```python
from build123d import *

# Parameters (mm, degrees)
BOSS_EXTRU_1_DEPTH      = 120
ENL_V_MAT_EXTRU_1_DEPTH = 188.009777727
ENL_V_MAT_EXTRU_2_DEPTH = 180.784310366
ESQUISSE6_R             = 2
ENL_V_MAT_EXTRU_3_DEPTH = 188.009777727
ESQUISSE7_R             = 2
ENL_V_MAT_EXTRU_4_DEPTH = 180.784310366
ESQUISSE10_R            = 1.364499713
ENL_V_MAT_EXTRU_5_DEPTH = 180.784310366
ENL_V_MAT_EXTRU_6_DEPTH = 188.009777727
ESQUISSE11_R            = 2
ENL_V_MAT_EXTRU_7_DEPTH = 188.009777727
ESQUISSE12_R            = 2
ENL_V_MAT_EXTRU_8_DEPTH = 180.784310366


with BuildPart() as part:
    # Esquisse3 → Boss.-Extru.1 (new body)
    with BuildSketch(Plane(origin=(0, 0, 0), x_dir=(1, 0, 0), z_dir=(0, 1, 0))):
        with BuildLine():
            ThreePointArc((-25, -28.618176043), (-27.104360033, -26.633694209), (-29.051678093, -24.494897428))
            Line((-29.051678093, -24.494897428), (-115, -24.494897428))
            Line((-115, -24.494897428), (-115, -28.618176043))
            Line((-115, -28.618176043), (-25, -28.618176043))
        make_face()
        with BuildLine():
            ThreePointArc((-10.103808925, -33.509894736), (-18.121448463, -29.943498553), (-25, -24.494897428))
            Line((-25, -24.494897428), (-29.051678093, -24.494897428))
            ThreePointArc((-29.051678093, -24.494897428), (-27.104360033, -26.633694209), (-25, -28.618176043))
            ThreePointArc((-25, -28.618176043), (-19.581111, -32.566548666), (-13.552631037, -35.50107311))
            ThreePointArc((-13.552631037, -35.50107311), (-10.809506446, -36.430132725), (-8.003591765, -37.147577564))
            Line((-8.003591765, -37.147577564), (-10.103808925, -33.509894736))
        make_face()
        with BuildLine():
            Line((35.411933246, -112.345472721), (-8.003591765, -37.147577564))
            ThreePointArc((-8.003591765, -37.147577564), (-10.809506446, -36.430132725), (-13.552631037, -35.50107311))
            Line((-13.552631037, -35.50107311), (31.963111135, -114.336651096))
            Line((31.963111135, -114.336651096), (35.411933246, -112.345472721))
        make_face()
    extrude(amount=BOSS_EXTRU_1_DEPTH)

    # Esquisse4 → Enlèv. mat.-Extru.1 (cut, through all)
    with BuildSketch(Plane.XY.offset(28.618176043)):
        with BuildLine():
            Line((-48, 105), (-48, 15))
            ThreePointArc((-48, 15), (-40, 7), (-32, 15))
            Line((-32, 15), (-32, 105))
            ThreePointArc((-32, 105), (-40, 113), (-48, 105))
        make_face()
    extrude(amount=-ENL_V_MAT_EXTRU_1_DEPTH, mode=Mode.SUBTRACT)

    # Esquisse5 → Enlèv. mat.-Extru.2 (cut, through all)
    with BuildSketch(Plane(origin=(-25.536888865, 0, 14.743729661), x_dir=(0.4999999999999999, 0, 0.8660254037844386), z_dir=(-0.8660254037844387, 0, 0.49999999999999994))):
        with BuildLine():
            Line((46.968515657, 105), (46.968515657, 15))
            ThreePointArc((46.968515657, 15), (38.968515657, 7), (30.968515657, 15))
            Line((30.968515657, 15), (30.968515657, 105))
            ThreePointArc((30.968515657, 105), (38.968515657, 113), (46.968515657, 105))
        make_face()
    extrude(amount=-ENL_V_MAT_EXTRU_2_DEPTH, mode=Mode.SUBTRACT)

    # Esquisse6 → Enlèv. mat.-Extru.3 (cut, through all)
    with BuildSketch(Plane.XY.offset(28.618176043)):
        with Locations((-110, 106.75)):
            Circle(ESQUISSE6_R)
    extrude(amount=-ENL_V_MAT_EXTRU_3_DEPTH, mode=Mode.SUBTRACT)

    # Esquisse7 → Enlèv. mat.-Extru.4 (cut, through all)
    with BuildSketch(Plane(origin=(-25.536888865, 0, 14.743729661), x_dir=(0.4999999999999999, 0, 0.8660254037844386), z_dir=(-0.8660254037844387, 0, 0.49999999999999994))):
        with Locations((110, 106.75)):
            Circle(ESQUISSE7_R)
    extrude(amount=-ENL_V_MAT_EXTRU_4_DEPTH, mode=Mode.SUBTRACT)

    # Esquisse10 → Enlèv. mat.-Extru.5 (cut, through all)
    with BuildSketch(Plane(origin=(-25.536888865, 0, 14.743729661), x_dir=(0.4999999999999999, 0, 0.8660254037844386), z_dir=(-0.8660254037844387, 0, 0.49999999999999994))):
        with Locations((101.5, 23.5)):
            Circle(ESQUISSE10_R)
        with Locations((52.5, 23.5)):
            Circle(ESQUISSE10_R)
        with Locations((52.5, 81.585512482)):
            Circle(ESQUISSE10_R)
        with Locations((101.5, 81.585512482)):
            Circle(ESQUISSE10_R)
    extrude(amount=-ENL_V_MAT_EXTRU_5_DEPTH, mode=Mode.SUBTRACT)

    # Esquisse9 → Enlèv. mat.-Extru.6 (cut, through all)
    with BuildSketch(Plane.XY.offset(28.618176043)):
        with BuildLine():
            ThreePointArc((-54.4, 23), (-56, 24.6), (-57.6, 23))
            ThreePointArc((-57.6, 23), (-56, 21.4), (-54.4, 23))
        make_face()
        with BuildLine():
            ThreePointArc((-106.1, 16.2), (-104.5, 14.6), (-102.9, 16.2))
            ThreePointArc((-102.9, 16.2), (-104.5, 17.8), (-106.1, 16.2))
        make_face()
        with BuildLine():
            ThreePointArc((-57.6, 98), (-56, 96.4), (-54.4, 98))
            ThreePointArc((-54.4, 98), (-56, 99.6), (-57.6, 98))
        make_face()
        with BuildLine():
            ThreePointArc((-106.1, 99), (-104.5, 97.4), (-102.9, 99))
            ThreePointArc((-102.9, 99), (-104.5, 100.6), (-106.1, 99))
        make_face()
    extrude(amount=-ENL_V_MAT_EXTRU_6_DEPTH, mode=Mode.SUBTRACT)

    # Esquisse11 → Enlèv. mat.-Extru.7 (cut, through all)
    with BuildSketch(Plane.XY.offset(28.618176043)):
        with Locations((-53, 13)):
            Circle(ESQUISSE11_R)
    extrude(amount=-ENL_V_MAT_EXTRU_7_DEPTH, mode=Mode.SUBTRACT)

    # Esquisse12 → Enlèv. mat.-Extru.8 (cut, through all)
    with BuildSketch(Plane(origin=(-25.536888865, 0, 14.743729661), x_dir=(0.4999999999999999, 0, 0.8660254037844386), z_dir=(-0.8660254037844387, 0, 0.49999999999999994))):
        with Locations((51.968515657, 13)):
            Circle(ESQUISSE12_R)
    extrude(amount=-ENL_V_MAT_EXTRU_8_DEPTH, mode=Mode.SUBTRACT)


solid = part.part
```
Read the model definition and answer for the solid it produces. Units are mm, in the model's axes. A direction names the side the tool comes from. Coordinates: 2 decimals unless noted, no trailing zeros. Order: outer loops, then holes, each group sorted by start corner. A loop starts at its lowest first (then second) coordinate and runs counter-clockwise, first axis right, second up. Notation, with made-up numbers: (31.25, 28) - (56.25, 28) arc R11 cw to (56.25, 46) - close; hole circle Ø3 at (63.5, 40). An arc over 180 degrees is marked (long way). Answer as a JSON object with one key per item and string values. Group by question number.
Item 1: Section B-B (y = 106.75) is taken. Give the vertices of the cut face in (x, z), plus the area to 3 significant figures.
Item 2: Flat-ended cylindrical pins translate along their axes: P1, Ø6.5, axis at x = -110, y = 106.75, coming from the -Z side; P2, Ø5, axis at x = -56, y = 98, coming from the +Z side; P3, Ø3.5, axis at y = 66, z = 27.5, coming from the +X side; P4, Ø10, axis at x = -18.5, y = 98, coming from the -Z side. Find the tip coordinate at first contact, or state that the pin passes through.
Item 3: Section D-D (z = 87) is taken. Give the vertices of the cut face in (x, y).
Item 4: Section C-C (x = 8) is taken. Give the vertices of the cut face in (y, z).
Item 5: Consider probe 1 along Y at (x, z) = (-104.5, 25.9); probe 2 along Y at (x, z) = (-56, 27.2); probe 3 along X at (y, z) = (98, 26). Determine where each line is inside the solid, lowest interval first. Write a range as from..to.
Item 6: Section A-A (y = 42) is taken. Give the vertices of the cut face in (x, z).
Item 7: A tool of negligible diameter and unlimited length cuts with its end or side. For faces 1 (the face through (-0.352, 60.63, 54.438)), 2 (the face through (-4.4, 113, 47.4)), 3 (the face through (-19.66, 59.16, 32.52)), 4 (the face through (-32, 59, 27)), from which of +Z, -Z, +X, -X, +Y, -Y can it reach the whole face along a straight path? Write none if from no direction.
Item 8: The mould has two halves that part along X. Classify faces 5 (the face through (-71, 59, 28.618)), 6 (the face through (-48, 61, 27)), 7 (the face through (-115, 59, 27)): +X half, -X half, draft (parallel to the pull), parting line (faces both ways), or undercut.
Results are:
{
 "1": {"outline": "(-115, 24.49) - (-112, 24.49) - (-112, 28.62) - (-115, 28.62) - close; (-108, 24.49) - (-47.81, 24.49) - (-47.81, 28.62) - (-108, 28.62) - close; (-32.19, 24.49) - (-25, 24.49) arc R35 cw to (-10.1, 33.51) - (-6.51, 39.74) - (-9.96, 41.73) - (-13.55, 35.5) arc R38 ccw to (-25, 28.62) - (-32.19, 28.62) - close; (-2.15, 55.25) - (1.3, 53.26) - (31.91, 106.28) - (28.46, 108.27) - close; (30.46, 111.74) - (33.91, 109.75) - (35.41, 112.35) - (31.96, 114.34) - close", "area": "621 mm^2"},
 "2": {"P1": "stops at z = 24.49", "P2": "stops at z = 28.62", "P3": "stops at x = -19.22", "P4": "stops at z = 25.94"},
 "3": {"outline": "(16.18, 0) - (20.78, 0) - (20.78, 120) - (16.18, 120) - close"},
 "4": {"outline": "(0, 64.87) - (120, 64.87) - (120, 72.83) - (0, 72.83) - close"},
 "5": {"probe 1": "y = 0..14.6, 17.8..97.4, 100.6..120", "probe 2": "y = 0..21.4, 24.6..96.4, 99.6..120", "probe 3": "x = -115..-105.75, -103.25..-57.6, -54.4..-48, -32..-23.43"},
 "6": {"outline": "(-115, 24.49) - (-48, 24.49) - (-48, 28.62) - (-115, 28.62) - close; (-32, 24.49) - (-25, 24.49) arc R35 cw to (-10.1, 33.51) - (-6.6, 39.57) - (-10.05, 41.56) - (-13.55, 35.5) arc R38 ccw to (-25, 28.62) - (-32, 28.62) - close; (-2.05, 55.42) - (1.4, 53.43) - (35.41, 112.35) - (31.96, 114.34) - close"},
 "7": {"face 1": "-Z, -X", "face 2": "none", "face 3": "+Z, -X, +Y, -Y", "face 4": "+Z, -Z"},
 "8": {"face 5": "draft", "face 6": "undercut", "face 7": "-X half"}
}
